Part print with two shaded views. Sizes in mm from the minimum x, y, z corner. Coordinates: 2 decimals unless noted, no trailing zeros. Loops run counter-clockwise (first coordinate to the right, second up) from the corner with the lowest first, then second, coordinate; pieces in that order, holes last. Notation, with made-up numbers: (-34.75, 61.25) - (-29.75, 61.25) arc R19 ccw to (-29.75, 76.25) - close; hole circle Ø6 at (55, 59). An arc over 180 degrees is marked (long way). Answer as CSV lines item,"result".
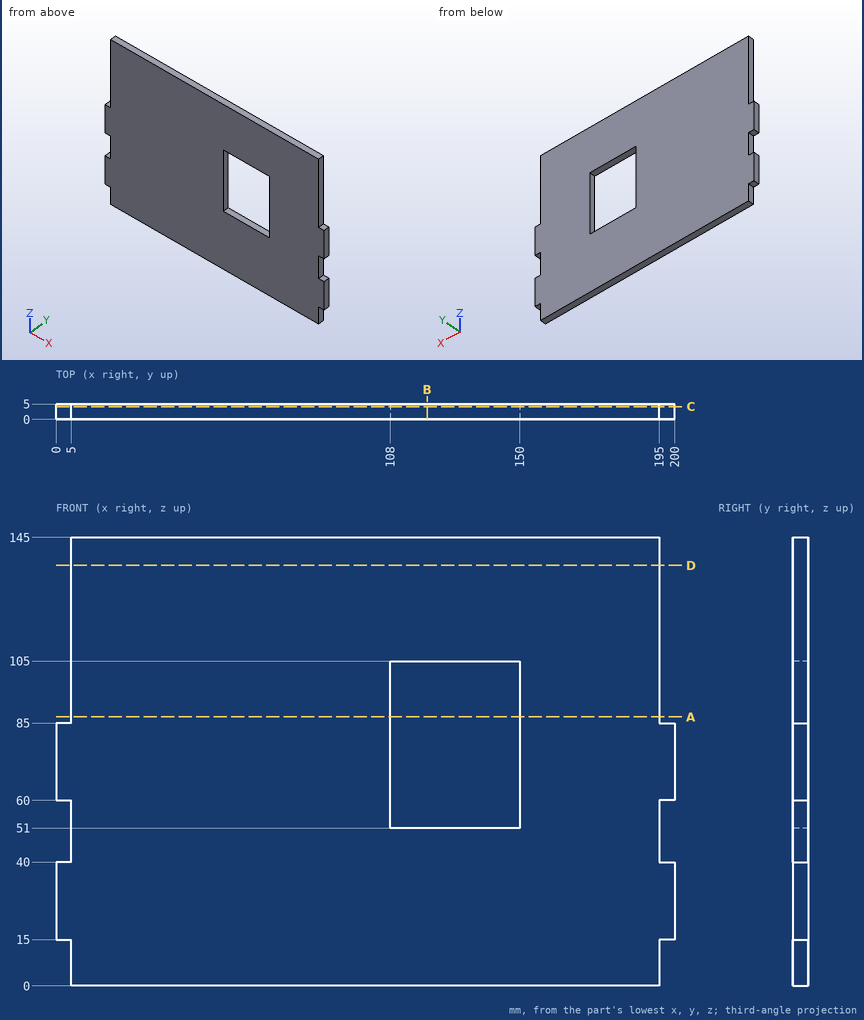
Q1. Saw through at B-B (x = 120). Give the cut face in (y, z), then the cut area to 3 significant figures.
Results:
outline,"(0, 0) - (5, 0) - (5, 51) - (0, 51) - close; (0, 105) - (5, 105) - (5, 145) - (0, 145) - close"
area,"455 mm^2"
Q2. Saw through at A-A (z = 87). Give the cut face in (x, y), then the cut area to 3 significant figures.
Results:
outline,"(5, 0) - (108, 0) - (108, 5) - (5, 5) - close; (150, 0) - (195, 0) - (195, 5) - (150, 5) - close"
area,"740 mm^2"
Q3. Saw through at D-D (z = 136). Give the cut face in (x, y), then the cut area to 3 significant figures.
Results:
outline,"(5, 0) - (195, 0) - (195, 5) - (5, 5) - close"
area,"950 mm^2"
Q4. Saw through at C-C (y = 4.15). Give the cut face in (x, z), then the cut area to 3 significant figures.
Results:
outline,"(0, 15) - (5, 15) - (5, 0) - (195, 0) - (195, 15) - (200, 15) - (200, 40) - (195, 40) - (195, 60) - (200, 60) - (200, 85) - (195, 85) - (195, 145) - (5, 145) - (5, 85) - (0, 85) - (0, 60) - (5, 60) - (5, 40) - (0, 40) - close; hole (108, 51) - (150, 51) - (150, 105) - (108, 105) - close"
area,"25,800 mm^2"
Q5. Wall check: L1, parallel to X at y = 1.65, z = 55.5; L2, parallel to X at y = 1.8, z = 65.5; L3, parallel to Z at x = 148.5, y = 2.5. Give the ranges that are in metal, low to high.
Results:
L1,"x = 5 to 108, 150 to 195"
L2,"x = 0 to 108, 150 to 200"
L3,"z = 0 to 51, 105 to 145"
Q6. Flat gauge pins, fed straight in: pin 1 (1.5 mm diameter, centred on y = 3, z = 7.5, fed in from -X); pin 2 (2.5 mm diameter, centred on x = 196.5, y = 3.5, fed in from -Z); pin 3 (2.5 mm diameter, centred on x = 2, y = 3, fed in from +Z). Where does each tip first touch, or does it go through?
Results:
pin 1,"stops at x = 5"
pin 2,"stops at z = 15"
pin 3,"stops at z = 85"
